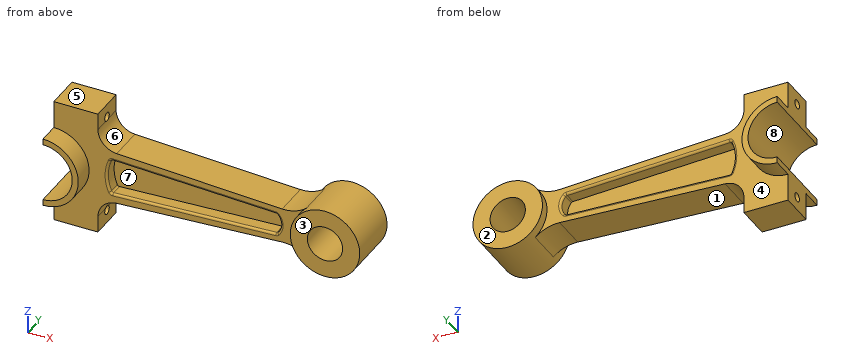
```python
from build123d import *

# Parameters (mm, degrees)
BOSS_EXTRUDE1_DEPTH = 16
SKETCH1_5_R         = 31.5
SKETCH1_5_R_2       = 16
BOSS_EXTRUDE2_DEPTH = 24
BOSS_EXTRUDE3_DEPTH = 35
CUT_EXTRUDE1_DEPTH  = 12
FILLET1_R           = 2
FILLET3_R           = 2
SKETCH6_R           = 4
CUT_EXTRUDE4_DEPTH  = 290.336969647


with BuildPart() as part:
    # Sketch1 → Boss-Extrude1 (new, symmetric)
    with BuildSketch(Plane(origin=(0, 0, 0), x_dir=(1, 0, 0), z_dir=(0, 1, 0))):
        with BuildLine():
            Line((-19.774827182, 56.996771876), (-19.774827182, 32))
            ThreePointArc((-19.774827182, 32), (12.225172818, 0), (-19.774827182, -32))
            Line((-19.774827182, -32), (-19.774827182, -56.996771876))
            Line((-19.774827182, -56.996771876), (20.225172818, -56.996771876))
            Line((20.225172818, -56.996771876), (20.225172818, -41.996771876))
            ThreePointArc((20.225172818, -41.996771876), (25.16884807, -29.597039719), (37.287694094, -24))
            Line((37.287694094, -24), (187.287694094, -16))
            ThreePointArc((187.287694094, -16), (199.120008212, -17.668601393), (209.448964206, -23.676975223))
            ThreePointArc((209.448964206, -23.676975223), (198.725172818, 0), (209.448964206, 23.676975223))
            ThreePointArc((209.448964206, 23.676975223), (199.120008212, 17.668601393), (187.287694094, 16))
            Line((187.287694094, 16), (37.287694094, 24))
            ThreePointArc((37.287694094, 24), (25.16884807, 29.597039719), (20.225172818, 41.996771876))
            Line((20.225172818, 41.996771876), (20.225172818, 56.996771876))
            Line((20.225172818, 56.996771876), (-19.774827182, 56.996771876))
        make_face()
    extrude(amount=BOSS_EXTRUDE1_DEPTH, both=True)

    # Sketch1_5 → Boss-Extrude2 (add, symmetric)
    with BuildSketch(Plane(origin=(0, 0, 0), x_dir=(1, 0, 0), z_dir=(0, 1, 0))):
        with Locations(Location((230.225172818, 0, 0), (0, 0, 270))):
            Circle(SKETCH1_5_R)
        with Locations(Location((230.225172818, 0, 0), (0, 0, 270))):
            Circle(SKETCH1_5_R_2, mode=Mode.SUBTRACT)
    extrude(amount=BOSS_EXTRUDE2_DEPTH, both=True)

    # Sketch1_6 → Boss-Extrude3 (add, symmetric)
    with BuildSketch(Plane(origin=(0, 0, 0), x_dir=(1, 0, 0), z_dir=(0, 1, 0))):
        with BuildLine():
            Line((-19.774827182, 32), (-19.774827182, 26.5))
            ThreePointArc((-19.774827182, 26.5), (6.725172818, 0), (-19.774827182, -26.5))
            Line((-19.774827182, -26.5), (-19.774827182, -32))
            ThreePointArc((-19.774827182, -32), (12.225172818, 0), (-19.774827182, 32))
        make_face()
    extrude(amount=BOSS_EXTRUDE3_DEPTH, both=True)

    # Sketch4 → Cut-Extrude1 (cut)
    with BuildSketch(Plane(origin=(0, 16, 0), x_dir=(1, 0, 0), z_dir=(0, 1, 0))):
        with BuildLine():
            Line((32.225172818, -16.001877998), (182.225172818, -9.501877998))
            ThreePointArc((182.225172818, -9.501877998), (186.160979553, 0), (182.225172818, 9.501877998))
            Line((182.225172818, 9.501877998), (32.225172818, 16.001877998))
            ThreePointArc((32.225172818, 16.001877998), (28.665381057, 0), (32.225172818, -16.001877998))
        make_face()
    cut_extrude1 = extrude(amount=-CUT_EXTRUDE1_DEPTH, mode=Mode.SUBTRACT)

    # Fillet1
    fillet1_edges = [part.edges().sort_by_distance(p)[0] for p in [
        (32.225172818, 10, 16.001877998),
        (32.225172818, 10, -16.001877998),
        (182.225172818, 10, -9.501877998),
        (182.225172818, 10, 9.501877998),
        (28.665381057, 16, 0),
        (107.225172818, 16, 12.751877998),
        (186.160979553, 16, 0),
        (107.225172818, 16, -12.751877998),
    ]]
    fillet(fillet1_edges, radius=FILLET1_R)

    # Mirror5: Cut-Extrude1 across plane
    add(cut_extrude1.mirror(Plane.ZX), mode=Mode.SUBTRACT)

    # Fillet3
    fillet3_edges = [part.edges().sort_by_distance(p)[0] for p in [
        (28.665381057, -16, 0),
        (32.225172818, -10, -16.001877998),
        (107.225172818, -16, 12.751877998),
        (32.225172818, -10, 16.001877998),
        (186.160979553, -16, 0),
        (182.225172818, -10, 9.501877998),
        (107.225172818, -16, -12.751877998),
        (182.225172818, -10, -9.501877998),
    ]]
    fillet(fillet3_edges, radius=FILLET3_R)

    # Sketch6 → Cut-Extrude4 (cut, through all)
    with BuildSketch(Plane.ZY.offset(19.774827182)):
        with Locations((-45, 0)):
            Circle(SKETCH6_R)
        with Locations(Location((45, 0, 0), (0, 0, 138.660333847))):
            Circle(SKETCH6_R)
    extrude(amount=-CUT_EXTRUDE4_DEPTH, mode=Mode.SUBTRACT)


solid = part.part
```
The listing builds one solid part. Answer for the finished solid, in the listing's coordinates (mm). Face numbers are marked on the shaded views. A direction names the side the tool comes from. Round coordinates to 2 decimals unless told otherwise and drop trailing zeros. Write each loop counter-clockwise with the first axis right and the second up, starting at its lowest first coordinate (ties: lowest second). Pieces come first, ordered by that corner, then holes. Notation, with made-up numbers: (58, 11) -> (73, 11) arc R15 cw to (73, 39) -> close; hole circle Ø7 at (42, 25.5). An arc over 180 degrees is marked (long way). Answer as a JSON object with one key per item and string values. Group by question number.
Q1. Section C-C (y = 20.5) is taken. Write down the section's boundary in (x, z), plus the area to 3 significant figures.
Q2. Determine the mould class of the marked faces 5, 6, 7 and 8 for opening direction X: pulls with the +X half, pulls with the -X half, needs draft (parallel to the pull), parting line crosses it, or undercut.
Q3. Section A-A (y = 0) is taken. Write down the section's boundary in (x, z).
Q4. Straight lines are drawn through the part: line 1 along Z through (x, y) = (8, 0); line 2 along Y through (x, z) = (6, -45); line 3 along Z through (x, y) = (4, 0). For each, find the intervals that lie inside material, in ascending order.
Q5. Section D-D (z = -45) is taken. Write down the section's boundary in (x, y).
Q6. Section B-B (z = 0) is taken. Write down the section's boundary in (x, y).
Q7. Each of these flat-tipped pins is pushed along its axis until it touches: pin 1 Ø16 at (x, z) = (69, -2.5) entering from +Y; pin 2 Ø7.5 at (y, z) = (7.5, 53) entering from +X; pin 3 Ø9 at (y, z) = (0, 45) entering from +X. Where does it stop, or does it pass through?
Q8. Which of the six approach directions +Z, -Z, +X, -X, +Y, -Y give full straight-line access (tool end or side, diameter ignored) to the marked faces 1, 2, 3 and 4?
Check values:
{
 "1": {"outline": "(-19.77, -32) arc R32 ccw to (-19.77, 32) -> (-19.77, 26.5) arc R26.5 cw to (-19.77, -26.5) -> close; circle Ø63 at (230.23, 0); hole circle Ø32 at (230.23, 0)", "area": "2,820 mm^2"},
 "2": {"face 5": "needs draft", "face 6": "undercut", "face 7": "undercut", "face 8": "pulls with the -X half"},
 "3": {"outline": "(-19.77, -57) -> (20.23, -57) -> (20.23, -49) -> (-19.77, -49) -> close; (-19.77, -41) -> (20.25, -41) arc R18.02 cw to (37.29, -24) -> (187.29, -16) arc R31.09 cw to (209.45, -23.68) arc R31.5 ccw (long way) to (209.45, 23.68) arc R31.09 cw to (187.29, 16) -> (37.29, 24) arc R18.02 cw to (20.25, 41) -> (-19.77, 41) -> (-19.77, 26.5) arc R26.5 cw to (-19.77, -26.5) -> close; (-19.77, 49) -> (20.23, 49) -> (20.23, 57) -> (-19.77, 57) -> close; hole circle Ø32 at (230.23, 0)"},
 "4": {"line 1": "-57 to -49, -41 to 41, 49 to 57", "line 2": "-16 to -4, 4 to 16", "line 3": "-57 to -49, -41 to -11.71, 11.71 to 41, 49 to 57"},
 "5": {"outline": "(-19.77, -16) -> (20.23, -16) -> (20.23, -4) -> (-19.77, -4) -> close; (-19.77, 4) -> (20.23, 4) -> (20.23, 16) -> (-19.77, 16) -> close"},
 "6": {"outline": "(6.73, -35) -> (12.23, -35) -> (12.23, -16) -> (26.67, -16) arc R2 ccw to (28.67, -14) -> (28.67, -4) -> (186.16, -4) -> (186.16, -14) arc R2 ccw to (188.16, -16) -> (198.73, -16) -> (198.73, -24) -> (214.23, -24) -> (214.23, 24) -> (198.73, 24) -> (198.73, 16) -> (188.16, 16) arc R2 ccw to (186.16, 14) -> (186.16, 4) -> (28.67, 4) -> (28.67, 14) arc R2 ccw to (26.67, 16) -> (12.23, 16) -> (12.23, 35) -> (6.73, 35) -> close; (246.23, -24) -> (261.73, -24) -> (261.73, 24) -> (246.23, 24) -> close"},
 "7": {"pin 1": "y = 4", "pin 2": "x = 20.23", "pin 3": "x = 20.29"},
 "8": {"face 1": "-Z, +Y, -Y", "face 2": "+Z, -Z, +X, +Y", "face 3": "+Z, -Z, +X, -Y", "face 4": "+Y"}
}
